Verification items for the finished model (mm, model axes). Coordinates: 2 decimals unless noted, no trailing zeros. Order: outer loops, then holes, each group sorted by start corner. A loop starts at its lowest first (then second) coordinate and runs counter-clockwise, first axis right, second up. Notation, with made-up numbers: M 11,-21.5 L 55,-21.5 A30 ccw 55,3.5 Z; hole C -1.5,57 d1. An arc over 180 degrees is marked long. Return JSON: item names as keys, results as strings. Group by question number.
1. Gauge pin test, flat ends, axial feed: pin 1 (1.5 mm diameter, centred on x = 7, y = -1, fed in from -Z); pin 2 (0.7 mm diameter, centred on x = 5, z = 0, fed in from +Y). Record the tip position at first contact, or that the pin passes through.
2. Material ranges on line 1 along Y through (x, z) = (0, 0.05); line 2 along X through (y, z) = (-0.5, -0.3); line 3 along X through (y, z) = (-0.3, 0.05), recorded low to high.
3. Section check A-A, the plane x = 3. Record the cut outline in (y, z), plus the area to 3 significant figures.
4. Mould release check, pull along Y, two halves, no side actions. Record for faces 1 (the cylindrical face through (1.1, 0.14, 0.01)), 2 (the cylindrical face through (8.1, -0.7, 0)), 3 (the cylindrical face through (-0.71, 0.02, 0.01)), 4 (the cylindrical face through (6.7, 0.7, 0)): +Y half, -Y half, draft (parallel to the pull), parting line (faces both ways), or undercut.
```python
from build123d import *

# Parameters (mm, degrees)
CUT_EXTRUDE_1_DEPTH      = 15.385405814
CUT_EXTRUDE_1_DEPTH_BACK = 15.385405814


with BuildPart() as part:
    # 扫描2: sweep along a path in Sketch 200
    with BuildLine(Plane.XY) as sweep_2_path:
        Line((11.8, 0.7), (1.8, 0.7))
        ThreePointArc((1.8, 0.7), (1.34176437, 0.785965522), (0.945844504, 1.032171582))
        ThreePointArc((0.945844504, 1.032171582), (-1.4, 0), (0.945844504, -1.032171582))
        ThreePointArc((0.945844504, -1.032171582), (1.34176437, -0.785965522), (1.8, -0.7))
        Line((1.8, -0.7), (14.3, -0.7))
    # 草图2 → 扫描2 (sweep)
    with BuildSketch(Plane(origin=(11.8, 0.7, 0), x_dir=(0, 0, 1), z_dir=(-1, 0, 0))):
        with BuildLine():
            Line((-0.699928568, -0.69), (0.699928568, -0.69))
            ThreePointArc((0.699928568, -0.69), (0, 0), (-0.699928568, -0.69))
        make_face()
    sweep(path=sweep_2_path.line)

    # 草图3 → 切除-拉伸1 (cut, two sides: drawn at the far end of the back side and taken through both)
    with BuildSketch(Plane.XY.offset(-CUT_EXTRUDE_1_DEPTH_BACK)):
        Polygon((11.8, 0.345), (11.303649235, 0.7), (14.31, 0.7), (14.31, -0.7), (13.79664716, -0.7), (14.3, -0.355), (13.803649235, 0), (11.29664716, 0), align=None)
    extrude(amount=CUT_EXTRUDE_1_DEPTH + CUT_EXTRUDE_1_DEPTH_BACK, mode=Mode.SUBTRACT)


solid = part.part
```
Answers follow:
{
 "1": {"pin 1": "z = -0.65", "pin 2": "y = 0.7"},
 "2": {"line 1": "-1.4 to -0.71, 0.71 to 1.4", "line 2": "-1.24 to -0.5, 0.51 to 14.09", "line 3": "-1.37 to -0.64, 0.78 to 14.22"},
 "3": {"outline": "M -0.01,-0.7 L -0.01,0.7 A0.7 ccw Z; M 0.01,-0.7 A0.7 ccw 0.01,0.7 Z", "area": "1.51 mm^2"},
 "4": {"face 1": "undercut", "face 2": "-Y half", "face 3": "undercut", "face 4": "+Y half"}
}
